Autodesk Inventor part; units mm, degrees
ref_plane "YZ Plane" through (0, 0, 0) normal (1, 0, 0) x (0, 1, 0)
ref_plane "XZ Plane" through (0, 0, 0) normal (0, 1, 0) x (-1, 0, 0)
ref_plane "XY Plane" through (0, 0, 0) normal (0, 0, 1) x (1, 0, 0)
sketch "スケッチ1" plane through (0, 0, 0) normal (0, 1, 0) x (-1, 0, 0)
  line L0 (0, 0) -> (-90, 0)
  line L1 (-90, 0) -> (-90, 50)
  line L2 (0, 50) -> (0, 0)
  line L3 (0, 0) -> (-5, 0)
  line L4 (-5, 0) -> (-5, 50)
  line L5 (-5, 0) -> (-90, 0)
  line L6 (-90, 0) -> (-85, 0)
  line L7 (-85, 0) -> (-85, 50)
  arc A0 (-85, 50) -> (-5, 50) centre (-45, 50) ccw
  line L8 (0, 0) -> (0, 10)
  line L9 (0, 10) -> (-90, 10)
  circle A1 centre (-45, 50) radius 45
  line L10 (-90, 5) -> (0, 5)
  line L11 (-90, 50) -> (-85, 50)
  line L12 (-5, 50) -> (0, 50)
  line L13 (0, 0) -> (-90, 0)
  line L14 (-90, 0) -> (-90, 5)
  line L15 (-90, 5) -> (0, 5)
  line L16 (0, 5) -> (0, 0)
  dimension "d0" = 90
  dimension "d1" = 50
  dimension "d2" = 5
  dimension "d3" = 85
  dimension "d4" = 5
  dimension "d5" = 80
  dimension "d6" = 10
  dimension "d7" = 90
extrude "押し出し1" add sketch "スケッチ1" along normal blind 230 contours L0 L4 L10 L2 | L0 L7 L10 L4 | L10 L4 L9 L2 | L0 L1 L10 L7 | L10 A1 L9 L4 | L9 L4 A1 L2 | L10 L1 L9 L7 | L7 L9 A1 L10 | L9 A1 L4 | A1 L9 | A1 L4 L12 | L9 L1 A1 L7 | L7 A1 L9 | A1 L9 A0 L4 | A1 L7 A0 L9 | L11 L7 A1
sketch "スケッチ2" plane through (0, 0, 0) normal (0, -1, 0) x (1, 0, 0)
  line L0 (0, 0) -> (0, 50)
  line L1 (90, 0) -> (0, 0)
  line L2 (90, 50) -> (90, 0)
  line L3 (85, 50) -> (90, 50)
  arc A0 (5, 50) -> (85, 50) centre (45, 50) ccw
  line L4 (0, 50) -> (5, 50)
  arc A1 (5, 23.467) -> (85, 23.467) centre (45, 50) ccw
  line L5 (0, 5) -> (90, 5)
  line L6 (5, 23.467) -> (5, 5)
  line L7 (85, 23.467) -> (85, 5)
  dimension "d29" = 48
extrude "押し出し2" cut sketch "スケッチ2" against normal blind 225 contours L6 A1 L5 | L5 A1 L7
sketch "スケッチ3" plane through (0, 230, 0) normal (0, 1, 0) x (1, 0, 0)
  arc A0 (85, -50) -> (5, -50) centre (45, -50) ccw
  line L0 (90, -50) -> (90, 0)
  line L1 (0, -50) -> (5, -50)
  arc A1 (85, -50) -> (5, -50) centre (45, -50) ccw
  line L2 (5, -50) -> (85, -50)
extrude "押し出し3" add sketch "スケッチ3" against normal blind 5
sketch "スケッチ4" plane through (90, 0, 50) normal (1, 0, 0) x (0, 0, -1)
  line L0 (0, 0) -> (50, 0)
  line L1 (0, 0) -> (0, 230)
  line L2 (25, 0) -> (25, 65)
  line L3 (25, 65) -> (25, 75)
  line L4 (25, 75) -> (25, 215)
  line L5 (25, 215) -> (25, 225)
  line L6 (0, 65) -> (40, 65)
  line L7 (40, 65) -> (40, 75)
  line L8 (40, 75) -> (0, 75)
  line L9 (0, 75) -> (0, 65)
  line L10 (0, 215) -> (40, 215)
  line L11 (40, 215) -> (40, 225)
  line L12 (40, 225) -> (0, 225)
  line L13 (0, 225) -> (0, 215)
  dimension "d16" = 65
  dimension "d17" = 10
  dimension "d18" = 140
  dimension "d19" = 10
  dimension "d20" = 40
extrude "押し出し4" cut sketch "スケッチ4" against normal blind 90 contours L1 L8 L3 L6 | L3 L8 L7 L6 | L1 L12 L5 L10 | L5 L12 L11 L10
sketch "スケッチ6" plane through (90, 0, 50) normal (1, 0, 0) x (0, 0, -1)
  line L0 (0, 230) -> (50, 230)
  line L1 (50, 230) -> (37.5, 251.6506)
  line L2 (50, 230) -> (110, 230) construction
  line L3 (0, 230) -> (37.5, 251.6506)
  line L4 (0, 230) -> (43.3013, 230) construction
  dimension "d32" = 120
  dimension "d33" = 30
extrude "押し出し6" add sketch "スケッチ6" against normal blind 90
sketch "スケッチ9" plane through (0, 0, 0) normal (-1, 0, 0) x (0, 0, 1)
  line L0 (10, 225) -> (50, 225)
  line L1 (50, 225) -> (50, 230)
  line L2 (50, 230) -> (12.5, 251.6506)
  line L3 (12.5, 251.6506) -> (0, 230)
  line L4 (0, 0) -> (0, 230)
  line L5 (0, 0) -> (50, 0)
  line L6 (50, 0) -> (50, 65)
  line L7 (50, 65) -> (10, 65)
  line L8 (10, 65) -> (10, 75)
  line L9 (10, 75) -> (50, 75)
  line L10 (50, 75) -> (50, 215)
  line L11 (50, 215) -> (10, 215)
  line L12 (10, 215) -> (10, 225)
  line L13 (12.5, 251.6506) -> (0, 230)
  line L14 (0, 230) -> (-132.7906, 0)
  line L15 (0, 145) -> (-49.0748, 145)
  line L16 (0, 115) -> (-66.3953, 115)
  dimension "d45" = 30
sketch "スケッチ10" plane through (0, 0, 0) normal (-1, 0, 0) x (0, 0, 1)
  line L0 (10, 225) -> (50, 225)
  line L1 (50, 225) -> (50, 230)
  line L2 (50, 230) -> (12.5, 251.6506)
  line L3 (12.5, 251.6506) -> (0, 230)
  line L4 (0, 0) -> (0, 230)
  line L5 (0, 0) -> (50, 0)
  line L6 (50, 0) -> (50, 65)
  line L7 (50, 65) -> (10, 65)
  line L8 (10, 65) -> (10, 75)
  line L9 (10, 75) -> (50, 75)
  line L10 (50, 75) -> (50, 215)
  line L11 (50, 215) -> (10, 215)
  line L12 (10, 215) -> (10, 225)
  line L13 (12.5, 251.6506) -> (-87.5, 78.4456)
  line L14 (-87.5, 78.4456) -> (50, 0)
sketch "スケッチ11" plane through (90, 230, 0) normal (0, 0.5, -0.866) x (-1, 0, 0)
  line L0 (0, 25) -> (90, 25)
  line L1 (45, 25) -> (45, 15)
  line L2 (45, 15) -> (60, 15)
  line L3 (60, 15) -> (30, 15)
  point P0 (90, -199.1858)
  dimension "d49" = 10
  dimension "d50" = 15
  dimension "d51" = 30
hole "穴1" at (45, 242.9904, 7.5) at (30, 242.9904, 7.5) at (60, 242.9904, 7.5) direction (0, -0.5, 0.866) diameter 2.5 depth 8 tip angle 118
sketch "スケッチ12" plane through (90, 0, 50) normal (1, 0, 0) x (0, 0, -1)
  line L0 (50, 0) -> (50, 230)
  line L1 (40, 225) -> (40, 215)
  line L2 (0, 215) -> (0, 75)
  line L3 (0, 145) -> (50, 145)
  line L4 (32.5, 175) -> (17.5, 175)
  line L5 (17.5, 175) -> (17.5, 115)
  line L6 (17.5, 115) -> (32.5, 115)
  line L7 (32.5, 115) -> (32.5, 175)
  line L8 (32.5, 175) -> (17.5, 115) construction
  line L9 (17.5, 175) -> (32.5, 115) construction
  line L10 (17.5, 145) -> (32.5, 145)
  line L11 (32.5, 145) -> (32.5, 115)
  line L12 (32.5, 115) -> (17.5, 115)
  line L13 (17.5, 115) -> (17.5, 145)
  point P0 (25, 145)
  dimension "d59" = 15
  dimension "d60" = 60
extrude "押し出し8" cut sketch "スケッチ12" against normal blind 2.5 contours L3 L7 L6 L5
sketch "スケッチ13" plane through (0, 0, 0) normal (-1, 0, 0) x (0, 0, 1)
  line L0 (0, 0) -> (0, 230)
  line L1 (50, 75) -> (50, 215)
  line L2 (50, 145) -> (0, 145)
  line L3 (17.5, 175) -> (32.5, 175)
  line L4 (32.5, 175) -> (32.5, 115)
  line L5 (32.5, 115) -> (17.5, 115)
  line L6 (17.5, 115) -> (17.5, 175)
  line L7 (17.5, 175) -> (32.5, 115) construction
  line L8 (32.5, 175) -> (17.5, 115) construction
  line L9 (17.5, 145) -> (32.5, 145)
  line L10 (32.5, 145) -> (32.5, 115)
  line L11 (32.5, 115) -> (17.5, 115)
  line L12 (17.5, 115) -> (17.5, 145)
  point P0 (25, 145)
  dimension "d63" = 15
  dimension "d64" = 60
extrude "押し出し9" cut sketch "スケッチ13" against normal blind 2.5 contours L4 L5 L6 L2
sketch "スケッチ14" plane through (90, 0, 0) normal (0, 0, -1) x (-1, 0, 0)
  line L0 (90, 0) -> (90, 230)
  line L1 (0, 0) -> (0, 230)
  line L2 (0, 145) -> (90, 145)
  line L3 (37.5, 175) -> (52.5, 175)
  line L4 (52.5, 175) -> (52.5, 115)
  line L5 (52.5, 115) -> (37.5, 115)
  line L6 (37.5, 115) -> (37.5, 175)
  line L7 (37.5, 175) -> (52.5, 115) construction
  line L8 (52.5, 175) -> (37.5, 115) construction
  line L9 (37.5, 145) -> (52.5, 145)
  line L10 (52.5, 145) -> (52.5, 175)
  line L11 (52.5, 175) -> (37.5, 175)
  line L12 (37.5, 175) -> (37.5, 145)
  point P0 (45, 145)
  dimension "d67" = 15
  dimension "d70" = 30
extrude "押し出し10" cut sketch "スケッチ14" against normal blind 2.5 contours L6 L3 L4 L2
sketch "スケッチ16" plane through (90, 0, 0) normal (0, 0, -1) x (-1, 0, 0)
  line L0 (52.5, 175) -> (52.5, 145)
  line L1 (52.5, 145) -> (37.5, 145)
  line L2 (37.5, 145) -> (37.5, 175)
  line L3 (90, 0) -> (90, 230)
  line L4 (0, 0) -> (0, 230)
  line L5 (0, 145) -> (90, 145)
  line L6 (0, 160) -> (37.5, 160)
  line L7 (52.5, 160) -> (90, 160)
  line L8 (18.75, 160) -> (18.75, 145)
  line L9 (71.25, 145) -> (71.25, 160)
  line L10 (11.25, 175) -> (26.25, 175)
  line L11 (26.25, 175) -> (26.25, 115)
  line L12 (26.25, 115) -> (11.25, 115)
  line L13 (11.25, 115) -> (11.25, 175)
  line L14 (11.25, 175) -> (26.25, 115) construction
  line L15 (26.25, 175) -> (11.25, 115) construction
  line L16 (11.25, 115) -> (26.25, 115)
  line L17 (26.25, 115) -> (26.25, 175)
  line L18 (26.25, 175) -> (11.25, 175)
  line L19 (11.25, 175) -> (11.25, 115)
  line L20 (45, 145) -> (45, 125)
  line L21 (78.75, 175) -> (63.75, 175)
  line L22 (63.75, 115) -> (78.75, 115)
  line L23 (78.75, 175) -> (78.75, 115)
  line L24 (63.75, 115) -> (63.75, 175)
  line L25 (63.75, 175) -> (78.75, 175)
  line L26 (78.75, 175) -> (78.75, 115)
  line L27 (78.75, 115) -> (63.75, 115)
  line L28 (63.75, 115) -> (63.75, 175)
  line L29 (11.25, 115) -> (26.25, 115)
  line L30 (26.25, 115) -> (26.25, 175)
  line L31 (26.25, 175) -> (11.25, 175)
  line L32 (11.25, 175) -> (11.25, 115)
  dimension "d71" = 15
  dimension "d72" = 60
  dimension "d73" = 20
extrude "押し出し11" cut sketch "スケッチ16" against normal blind 3 contours L24 L21 L23 L7 | L7 L9 L5 L24 | L5 L23 L22 L24 | L7 L23 L5 L9 | L11 L12 L13 L5 | L5 L8 L6 L11 | L6 L13 L10 L11 | L5 L13 L6 L8
sketch "スケッチ17" plane through (37.5, 145, 0) normal (0, 1, 0) x (1, 0, 0)
  line L0 (-57.7643, 16.522) -> (69.053, 16.522)
  line L1 (69.053, 16.522) -> (69.053, -65.9751)
  line L2 (69.053, -65.9751) -> (-57.7643, -65.9751)
  line L3 (-57.7643, -65.9751) -> (-57.7643, 16.522)
  point P0 (-37.5, 0)
extrude "押し出し12" cut sketch "スケッチ17" along normal blind 120
sketch "スケッチ18" plane through (90, 0, 0) normal (0, 0, -1) x (-1, 0, 0)
  line L0 (63.75, 145) -> (26.25, 145)
  line L1 (37.5, 170) -> (52.5, 170)
  line L2 (52.5, 170) -> (52.5, 120)
  line L3 (52.5, 120) -> (37.5, 120)
  line L4 (37.5, 120) -> (37.5, 170)
  line L5 (37.5, 170) -> (52.5, 120) construction
  line L6 (52.5, 170) -> (37.5, 120) construction
  point P0 (45, 145)
  dimension "d78" = 15
  dimension "d79" = 50
extrude "押し出し13" add sketch "スケッチ18" against normal blind 5
sketch "スケッチ19" plane through (0, 0, 0) normal (0, -1, 0) x (1, 0, 0)
  line L0 (0, 0) -> (0, 50)
  line L1 (90, 0) -> (0, 0)
  line L2 (90, 50) -> (90, 0)
  line L3 (85, 50) -> (90, 50)
  arc A0 (5, 50) -> (85, 50) centre (45, 50) ccw
  line L4 (0, 50) -> (5, 50)
  line L5 (-25.7833, 110.7871) -> (115.7833, 110.7871)
  line L6 (115.7833, 110.7871) -> (115.7833, -10.7871)
  line L7 (115.7833, -10.7871) -> (-25.7833, -10.7871)
  line L8 (-25.7833, -10.7871) -> (-25.7833, 110.7871)
  line L9 (-25.7833, 110.7871) -> (115.7833, -10.7871) construction
  line L10 (115.7833, 110.7871) -> (-25.7833, -10.7871) construction
extrude "押し出し14" cut sketch "スケッチ19" against normal blind 40 contours L0 L4 A0 L3 L2 L1 | L5 L6 L7 L8
properties part number "知能ロボコン発射台２.2" material "ABS プラスチック"
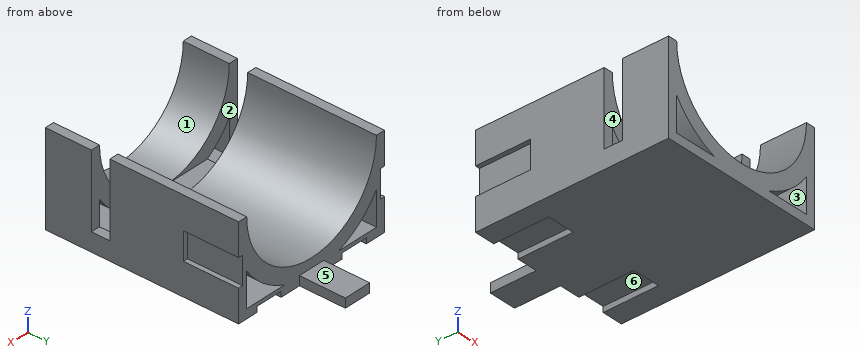
Read the model definition and answer for the solid it produces. Units are mm, in the model's axes. Face numbers are marked on the shaded views. A direction names the side the tool comes from. Give positions to 0.01 mm unless a question says otherwise; leave off trailing zeros. Write each loop counter-clockwise with the first axis right and the second up, starting at its lowest first coordinate (ties: lowest second). Pieces come first, ordered by that corner, then holes. Notation, with made-up numbers: (-26.75, -9) -> (-9.75, -9) arc R7 cw to (-9.75, -3) -> close; hole circle Ø3 at (6, 38). An arc over 180 degrees is marked (long way). Answer as a JSON object with one key per item and string values. Group by question number.
1) Find section D-D (z = 14). Count the separate pieces of the cut face and the enclosed holes in it, and give its area (3 significant figures).
2) Find section C-C (z = 41.5). Write down the section's boundary in (x, y).
3) Find section A-A (y = 54). Write down the section's boundary in (x, z), and give its area (3 significant figures).
4) Find section B-B (x = 14.5). Write down the section's boundary in (y, z).
5) Each of these flat-tipped pins is pushed along its axis until it touches: P1, Ø7.5, axis at y = 127, z = 22, coming from the -X side; P2, Ø7.5, axis at x = 21, y = 126, coming from the -Z side; P3, Ø8, axis at x = 57, y = 83.5, coming from the +Z side. Where does it stop, or does it pass through?
6) Consider L1, parallel to X at y = 103, z = 17.5; L2, parallel to X at y = 128, z = 14; L3, parallel to Z at x = 65, y = 137. Determine where each line is inside the solid, lowest interval first. Write a range as from..to.
7) A tool of negligible diameter and unlimited length cuts with its end or side. For the marked faces 4, 5 and 6, from which of +Z, -Z, +X, -X, +Y, -Y can it reach the whole face along a straight path? Write none if from no direction.
8) The mould has two halves that part along Z. Classify the marked faces 1, 2 and 3: +Z half, -Z half, draft (parallel to the pull), parting line (faces both ways), or undercut.
Values follow:
{
 "1": {"separate pieces": "8", "enclosed holes": "0", "area": "3,670 mm2"},
 "2": {"outline": "(0, 40) -> (5.91, 40) -> (5.91, 65) -> (0, 65) -> close; (0, 75) -> (5.91, 75) -> (5.91, 145) -> (0, 145) -> close; (84.09, 40) -> (90, 40) -> (90, 65) -> (84.09, 65) -> close; (84.09, 75) -> (90, 75) -> (90, 145) -> (84.09, 145) -> close"},
 "3": {"outline": "(0, 0) -> (90, 0) -> (90, 50) -> (85, 50) arc R40 cw to (5, 50) -> (0, 50) -> close; hole (5, 5) -> (28.3, 5) arc R48 cw to (5, 23.47) -> close; hole (61.7, 5) -> (85, 5) -> (85, 23.47) arc R48 cw to start", "area": "1,650 mm2"},
 "4": {"outline": "(40, 0) -> (115, 0) -> (115, 3) -> (145, 3) -> (145, 5) -> (40, 5) -> close; (40, 12.94) -> (65, 12.94) -> (65, 24.12) -> (40, 24.12) -> close; (75, 12.94) -> (145, 12.94) -> (145, 24.12) -> (75, 24.12) -> close"},
 "5": {"P1": "stops at x = 2.5", "P2": "stops at z = 3", "P3": "stops at z = 13.34"},
 "6": {"L1": "x = 0..5, 9.68..21.68, 68.32..80.32, 85..90", "L2": "x = 0..5, 13.25..27.56, 62.44..76.75, 85..90", "L3": "z = 3..5, 6.37..15.36"},
 "7": {"face 4": "+Z, +X, -X", "face 5": "+Z, +X, -X, +Y", "face 6": "-Z, +Y"},
 "8": {"face 1": "+Z half", "face 2": "draft", "face 3": "undercut"}
}
